Could you check a few things on this model? Use its own coordinates, in mm. Face numbers are marked on the shaded views. A direction names the side the tool comes from. Coordinates: 2 decimals unless noted, no trailing zeros. Write each loop counter-clockwise with the first axis right and the second up, starting at its lowest first coordinate (ties: lowest second). Pieces come first, ordered by that corner, then holes. Notation, with made-up numbers: M 2,21.5 L 40,21.5 A18 ccw 40,31.5 Z; hole C 27.5,57.5 d5. An arc over 180 degrees is marked long. Answer as CSV lines item,"result". Start each with the question number.
Item 1: We'd pull the mould along X, two halves only. Please class the marked faces 1, 2 and 3: +X half, -X half, draft (parallel to the pull), parting line (faces both ways), or undercut.
Item 2: Suppose I cut it at D-D, the plane x = -27. Write out the boundary of the cut face in (y, z), and give its area (3 significant figures).
Item 3: If I drill on line 1 along X through (y, z) = (-102.5, -39.5); line 2 along Y through (x, z) = (8, 28); line 3 along X through (y, z) = (-120, -34), over which ranges is the centre line in solid material (lowest first)? Write a range as [from, to].
Item 4: Suppose I cut it at A-A, the plane x = 12.5. Write out the boundary of the cut face in (y, z), and give its area (3 significant figures).
Item 5: On a 3-axis mill with a long thin cutter (end or side, diameter ignored), from which of +Z, -Z, +X, -X, +Y, -Y can I reach the whole of each face in a straight line? I mean the marked faces 4, 5 and 6. Say none if no direction works.
Item 6: Suppose I cut it at C-C, the plane y = -17.5. Write out the boundary of the cut face in (x, z), and give its area (3 significant figures).
Item 7: I'm going to push flat-ended pins straight in: P1, Ø9.5, axis at x = -84.45, y = -103.3, coming from the -Z side; P2, Ø16, axis at y = -76.5, z = 31, coming from the +X side; P3, Ø4, axis at y = -41.5, z = 30.5, coming from the +X side; P4, Ø2, axis at y = -67.5, z = -13.5, coming from the +X side. Where does each tip first touch, or does it pass through?
Item 8: Suppose I cut it at B-B, the plane y = -74. Write out the boundary of the cut face in (x, z), and give its area (3 significant figures).
```python
from build123d import *

# Parameters (mm, degrees)
F0_W         = 203.2
F0_H         = 127
F1_DEPTH     = 127
F3_DEPTH     = 76.2
F4_SIZE2     = 101.6
F4_SIZE      = 76.2
F5_R         = 5.08
F6_T1_DEPTH  = 116.84
F6_T3_DEPTH  = 116.84
F6_T5_DEPTH  = 193.04
F6_S9_W      = 5.08
F6_S9_H      = 5.08
F6_T10_DEPTH = 5.08
F6_S15_W     = 5.08
F6_S15_H     = 5.08
F6_T16_DEPTH = 5.08
F6_S21_W     = 5.08
F6_S21_H     = 5.08
F6_T22_DEPTH = 5.08
F6_S27_W     = 5.08
F6_S27_H     = 5.08
F6_T28_DEPTH = 5.08
F7_R         = 18.4939106261
F8_DEPTH     = 50.8
F9_R         = 7.7650869993
F10_DEPTH    = 127


# Not quite as in the source:
# - a fillet or chamfer that OpenCascade refuses, or shapes differently, is made with other operations: its cross-section is extruded or revolved along the edge and cut away or added


with BuildPart() as f1:
    # F0 (on Front) → F1 (new body)
    with BuildSketch(Plane.XZ):
        Rectangle(F0_W, F0_H)
    extrude(amount=F1_DEPTH)

    # F2 (on face) → F3 (cut)
    with BuildSketch(Plane.XZ.offset(127)):
        Polygon((101.6, 63.5), (0, 63.5), (0, 0), (-35.8415916562, 0), (-35.8415916562, -63.5), (101.6, -63.5), align=None)
    extrude(amount=-F3_DEPTH, mode=Mode.SUBTRACT)

    # F4
    f4_edges = [f1.edges().sort_by_distance(p)[0] for p in [
        (101.6, -25.4, 63.5),
    ]]
    f4_side = f1.faces().sort_by_distance((-21.771429, -52.614286, 63.5))[0]
    chamfer(f4_edges, length=F4_SIZE, length2=F4_SIZE2, reference=f4_side)

    # F5
    f5_edges = [f1.edges().sort_by_distance(p)[0] for p in [
        (-101.6, -63.5, 63.5),
        (-50.8, -127, 63.5),
        (0, -88.9, 63.5),
        (12.7, -50.8, 63.5),
        (25.4, -25.4, 63.5),
        (-38.1, 0, 63.5),
        (-17.920796, -127, 0),
        (0, -88.9, 0),
        (-101.6, -127, 0),
        (-68.720796, -127, -63.5),
        (-35.841592, -88.9, -63.5),
        (-35.841592, -50.8, -31.75),
        (32.879204, -50.8, -63.5),
        (101.6, -50.8, -50.8),
        (101.6, -25.4, -63.5),
        (101.6, 0, -50.8),
        (101.6, -25.4, -38.1),
        (63.5, -50.8, 12.7),
        (63.5, 0, 12.7),
    ]]
    fillet(f5_edges, radius=F5_R)

    # F6: fillet of radius 5.08 on 3 edges, made by hand

    # F6_s2 → F6_t1 (cut)
    with BuildSketch(Plane.XZ.offset(5.08)):
        with BuildLine():
            ThreePointArc((-96.52, -63.5), (-100.1121024484, -62.0121024484), (-101.6, -58.42))
            Line((-101.6, -58.42), (-101.6, -63.5))
            Line((-101.6, -63.5), (-96.52, -63.5))
        make_face()
    extrude(amount=F6_T1_DEPTH, mode=Mode.SUBTRACT)

    # F6_s4 → F6_t3 (cut)
    with BuildSketch(Plane.XY.offset(-58.42)):
        with BuildLine():
            ThreePointArc((-96.52, 0), (-100.1121024484, -1.4878975516), (-101.6, -5.08))
            Line((-101.6, -5.08), (-101.6, 0))
            Line((-101.6, 0), (-96.52, 0))
        make_face()
    extrude(amount=F6_T3_DEPTH, mode=Mode.SUBTRACT)

    # F6_s6 → F6_t5 (cut)
    with BuildSketch(Plane.YZ.offset(-96.52)):
        with BuildLine():
            ThreePointArc((0, -58.42), (-1.4878975516, -62.0121024484), (-5.08, -63.5))
            Line((-5.08, -63.5), (0, -63.5))
            Line((0, -63.5), (0, -58.42))
        make_face()
    extrude(amount=F6_T5_DEPTH, mode=Mode.SUBTRACT)


with BuildPart() as f6_tool8:
    # F6_s9 → F6_t10 (new body)
    with BuildSketch(Plane.XZ.offset(5.08)):
        with Locations((99.06, -60.96)):
            Rectangle(F6_S9_W, F6_S9_H)
    extrude(amount=-F6_T10_DEPTH)

    # F6_s11 → F6_t12 (revolve, cut)
    with BuildSketch(Plane(origin=(96.52, -5.08, -58.42), x_dir=(-0.7071067812, 0, 0.7071067812), z_dir=(-0.7071067812, 0, -0.7071067812))):
        with BuildLine():
            ThreePointArc((0, -5.08), (5.08, 0), (0, 5.08))
            Line((0, 5.08), (0, -5.08))
        make_face()
    revolve(axis=Axis((96.52, -5.08, -58.42), (0, 1, 0)), mode=Mode.SUBTRACT)


with BuildPart() as f1_1:
    add(f1.part)

    # F6_t7: cut F6_tool8
    add(f6_tool8.part, mode=Mode.SUBTRACT)


with BuildPart() as f6_tool14:
    # F6_s15 → F6_t16 (new body)
    with BuildSketch(Plane.XZ.offset(5.08)):
        with Locations((-99.06, 60.96)):
            Rectangle(F6_S15_W, F6_S15_H)
    extrude(amount=-F6_T16_DEPTH)

    # F6_s17 → F6_t18 (revolve, cut)
    with BuildSketch(Plane(origin=(-96.52, -5.08, 58.42), x_dir=(0.7071067812, 0, -0.7071067812), z_dir=(0.7071067812, 0, 0.7071067812))):
        with BuildLine():
            ThreePointArc((0, -5.08), (5.08, 0), (0, 5.08))
            Line((0, 5.08), (0, -5.08))
        make_face()
    revolve(axis=Axis((-96.52, -5.08, 58.42), (0, 1, 0)), mode=Mode.SUBTRACT)


with BuildPart() as f1_2:
    add(f1_1.part)

    # F6_t13: cut F6_tool14
    add(f6_tool14.part, mode=Mode.SUBTRACT)


with BuildPart() as f6_tool20:
    # F6_s21 → F6_t22 (new body)
    with BuildSketch(Plane.XY.offset(-58.42)):
        with Locations((-99.06, -124.46)):
            Rectangle(F6_S21_W, F6_S21_H)
    extrude(amount=-F6_T22_DEPTH)

    # F6_s23 → F6_t24 (revolve, cut)
    with BuildSketch(Plane(origin=(-96.52, -121.92, -58.42), x_dir=(0.7071067812, 0.7071067812, 0), z_dir=(-0.7071067812, 0.7071067812, 0))):
        with BuildLine():
            ThreePointArc((0, -5.08), (5.08, 0), (0, 5.08))
            Line((0, 5.08), (0, -5.08))
        make_face()
    revolve(axis=Axis((-96.52, -121.92, -58.42), (0, 0, -1)), mode=Mode.SUBTRACT)


with BuildPart() as f1_3:
    add(f1_2.part)

    # F6_t19: cut F6_tool20
    add(f6_tool20.part, mode=Mode.SUBTRACT)


with BuildPart() as f6_tool26:
    # F6_s27 → F6_t28 (new body)
    with BuildSketch(Plane.XZ.offset(5.08)):
        with Locations((-99.06, -60.96)):
            Rectangle(F6_S27_W, F6_S27_H)
    extrude(amount=-F6_T28_DEPTH)

    # F6_s29 → F6_t30 (revolve, cut)
    with BuildSketch(Plane(origin=(-96.52, -5.08, -58.42), x_dir=(0.7071067812, 0, 0.7071067812), z_dir=(-0.7071067812, 0, 0.7071067812))):
        with BuildLine():
            ThreePointArc((0, -5.08), (5.08, 0), (0, 5.08))
            Line((0, 5.08), (0, -5.08))
        make_face()
    revolve(axis=Axis((-96.52, -5.08, -58.42), (0, 1, 0)), mode=Mode.SUBTRACT)


with BuildPart() as f1_4:
    add(f1_3.part)

    # F6_t25: cut F6_tool26
    add(f6_tool26.part, mode=Mode.SUBTRACT)

    # F7 (on face) → F8 (cut, through all)
    with BuildSketch(Plane.XZ.offset(50.8)):
        with Locations((18.6727233231, -28.0290115625)):
            Circle(F7_R)
    extrude(amount=-F8_DEPTH, mode=Mode.SUBTRACT)

    # F9 (on face) → F10 (cut, through all)
    with BuildSketch(Plane.XY.offset(63.5)):
        with Locations((-84.4542831182, -103.3027470112)):
            Circle(F9_R)
    extrude(amount=-F10_DEPTH, mode=Mode.SUBTRACT)


solid = f1_4.part
```
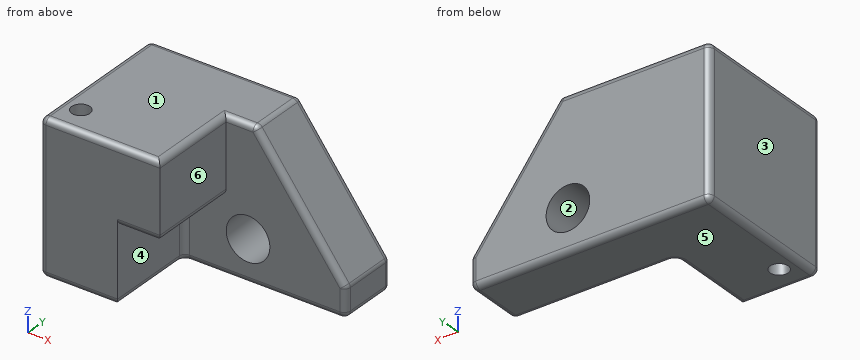
Ans:
1,face 1,"draft"
1,face 2,"undercut"
1,face 3,"-X half"
2,outline,"M -127,5.08 A5.08 ccw -121.92,0 L -50.8,0 L -50.8,-58.42 A5.08 ccw -45.72,-63.5 L -5.08,-63.5 A5.08 ccw 0,-58.42 L 0,58.42 A5.08 ccw -5.08,63.5 L -121.92,63.5 A5.08 ccw -127,58.42 Z"
2,area,"11,300 mm^2"
3,line 1,"x = [-101.6, -92.18], [-76.73, -35.84]"
3,line 2,"y = [-50.8, 0]"
3,line 3,"x = [-101.6, -35.84]"
4,outline,"M -50.8,-58.42 A5.08 ccw -45.72,-63.5 L -5.08,-63.5 A5.08 ccw 0,-58.42 L 0,-45.46 L -50.8,-45.46 Z; M -50.8,-10.6 L 0,-10.6 L 0,58.42 A5.08 ccw -5.08,63.5 L -45.72,63.5 A5.08 ccw -50.8,58.42 Z"
4,area,"4,660 mm^2"
5,face 4,"-Z, +X, -Y"
5,face 5,"-Z, +X, -X, +Y, -Y"
5,face 6,"+Z, -Z, +X, -Y"
6,outline,"M -101.6,-58.42 A5.08 ccw -96.52,-63.5 L 96.52,-63.5 A5.08 ccw 101.6,-58.42 L 101.6,-39.79 A5.08 ccw 100.58,-36.75 L 26.92,61.47 A5.08 ccw 22.86,63.5 L -96.52,63.5 A5.08 ccw -101.6,58.42 Z; hole C 18.67,-28.03 d36.99"
6,area,"20,800 mm^2"
7,P1,"passes through"
7,P2,"stops at x = 0"
7,P3,"stops at x = 51.65"
7,P4,"stops at x = -35.84"
8,outline,"M -101.6,-58.42 A5.08 ccw -96.52,-63.5 L -40.92,-63.5 A5.08 ccw -35.84,-58.42 L -35.84,0 L -5.08,0 A5.08 ccw 0,5.08 L 0,58.42 A5.08 ccw -5.08,63.5 L -96.52,63.5 A5.08 ccw -101.6,58.42 Z"
8,area,"10,600 mm^2"
